from build123d import *

# Parameters (mm, degrees)
F1_DEPTH = 25.4
F3_DEPTH = 25.401


with BuildPart() as f1:
    # F0 (on Front) → F1 (new body)
    with BuildSketch(Plane.XZ):
        with BuildLine():
            Line((170.549796, 190.5), (-69.162704, 190.5))
            ThreePointArc((-69.162704, 190.5), (-82.633088, 184.920384), (-88.212704, 171.45))
            Line((-88.212704, 171.45), (-88.212704, -44.45))
            ThreePointArc((-88.212704, -44.45), (-82.633088, -57.920384), (-69.162704, -63.5))
            Line((-69.162704, -63.5), (121.337296, -63.5))
            ThreePointArc((121.337296, -63.5), (134.80768, -57.920384), (140.387296, -44.45))
            Line((140.387296, -44.45), (140.387296, 98.425))
            ThreePointArc((140.387296, 98.425), (141.317232, 100.670064), (143.562296, 101.6))
            Line((143.562296, 101.6), (148.324796, 101.6))
            ThreePointArc((148.324796, 101.6), (150.56986, 100.670064), (151.499796, 98.425))
            Line((151.499796, 98.425), (151.499796, 12.7))
            ThreePointArc((151.499796, 12.7), (155.21954, 3.719744), (164.199796, 0))
            Line((164.199796, 0), (176.899796, 0))
            ThreePointArc((176.899796, 0), (185.880052, 3.719744), (189.599796, 12.7))
            Line((189.599796, 12.7), (189.599796, 171.45))
            ThreePointArc((189.599796, 171.45), (184.02018, 184.920384), (170.549796, 190.5))
        make_face()
    extrude(amount=F1_DEPTH)

    # F2 (on face) → F3 (cut, through all)
    with BuildSketch(Plane.XZ.offset(25.4)):
        with BuildLine():
            Line((64.187296, 165.1), (-24.712704, 165.1))
            ThreePointArc((-24.712704, 165.1), (-33.69296, 161.380256), (-37.412704, 152.4))
            Line((-37.412704, 152.4), (-37.412704, 146.05))
            ThreePointArc((-37.412704, 146.05), (-33.69296, 137.069744), (-24.712704, 133.35))
            Line((-24.712704, 133.35), (64.187296, 133.35))
            ThreePointArc((64.187296, 133.35), (73.167552, 137.069744), (76.887296, 146.05))
            Line((76.887296, 146.05), (76.887296, 152.4))
            ThreePointArc((76.887296, 152.4), (73.167552, 161.380256), (64.187296, 165.1))
        make_face()
    extrude(amount=-F3_DEPTH, mode=Mode.SUBTRACT)


solid = f1.part
Read the model definition and answer for the solid it produces. Units are mm, in the model's axes. A direction names the side the tool comes from. Round coordinates to 2 decimals unless told otherwise and drop trailing zeros. Loops run counter-clockwise (first coordinate to the right, second up) from the corner with the lowest first, then second, coordinate; pieces in that order, holes last.
Q1. Consider probe 1 along Z at (x, y) = (4.5, -13.25); probe 2 along X at (y, z) = (-7.5, 31); probe 3 along X at (y, z) = (-8.5, -6). Determine where each line is inside the solid, lowest interval first.
Q2. Section A-A on x = 50 is taken. Write down the section's boundary in (y, z).
Q3. Section D-D on z = -6 is taken. Write down the section's boundary in (x, y), and give its area (3 significant figures).
Q4. Determine the mould class of faces 1 (the face through (189.6, -13, 91)), 2 (the face through (20, -13, 165.1)), 3 (the face through (25, -13, -63.5)) for opening direction Z: released by +Z, released by -Z, zero draft, split by the parting line, or undercut.
Q5. Which of the six approach directions +Z, -Z, +X, -X, +Y, -Y give full straight-line access (tool end or side, diameter ignored) to faces 4 (the face through (170, -13, 0)), 5 (the face through (-33.59, -12.88, 161.48)), 6 (the face through (155.12, -12.52, 3.82)), 7 (the face through (49, -25.4, 65))?
Q6. Each of these flat-tipped pins is pushed along its axis until it touches: pin 1 (4 mm diameter, centred on x = 147, y = -11, fed in from -Z); pin 2 (14 mm diameter, centred on x = 171, y = -15.5, fed in from -Z). Where does it stop, or does it pass through?
Q7. Section C-C on y = -9 is taken. Write down the section's boundary in (x, z) (3 decimals).
Q8. Section B-B on z = 84 is taken. Write down the section's boundary in (x, y), and give its area (3 significant figures).
Output:
1. probe 1: z = -63.5 to 133.35, 165.1 to 190.5
1. probe 2: x = -88.21 to 140.39, 151.5 to 189.6
1. probe 3: x = -88.21 to 140.39
2. outline: (-25.4, -63.5) - (0, -63.5) - (0, 133.35) - (-25.4, 133.35) - close; (-25.4, 165.1) - (0, 165.1) - (0, 190.5) - (-25.4, 190.5) - close
3. outline: (-88.21, -25.4) - (140.39, -25.4) - (140.39, 0) - (-88.21, 0) - close
3. area: 5,810 mm2
4. face 1: zero draft
4. face 2: undercut
4. face 3: released by -Z
5. face 4: -Z, +X, +Y, -Y
5. face 5: +Y, -Y
5. face 6: -Z, +Y, -Y
5. face 7: +Z, -Z, +X, -X, -Y
6. pin 1: stops at z = 101.53
6. pin 2: stops at z = 0
7. outline: (-88.213, -44.45) arc R19.05 ccw to (-69.163, -63.5) - (121.337, -63.5) arc R19.05 ccw to (140.387, -44.45) - (140.387, 98.425) arc R3.175 cw to (143.562, 101.6) - (148.325, 101.6) arc R3.175 cw to (151.5, 98.425) - (151.5, 12.7) arc R12.7 ccw to (164.2, 0) - (176.9, 0) arc R12.7 ccw to (189.6, 12.7) - (189.6, 171.45) arc R19.05 ccw to (170.55, 190.5) - (-69.163, 190.5) arc R19.05 ccw to (-88.213, 171.45) - close; hole (-37.413, 146.05) arc R12.7 ccw to (-24.713, 133.35) - (64.187, 133.35) arc R12.7 ccw to (76.887, 146.05) - (76.887, 152.4) arc R12.7 ccw to (64.187, 165.1) - (-24.713, 165.1) arc R12.7 ccw to (-37.413, 152.4) - close
8. outline: (-88.21, -25.4) - (140.39, -25.4) - (140.39, 0) - (-88.21, 0) - close; (151.5, -25.4) - (189.6, -25.4) - (189.6, 0) - (151.5, 0) - close
8. area: 6,770 mm2
